```python
from build123d import *

# Parameters (mm, degrees)
BOSS_EXTRUDE1_DEPTH = 25
SKETCH2_R           = 2
CUT_EXTRUDE1_DEPTH  = 6
SKETCH3_R           = 2
CUT_EXTRUDE2_DEPTH  = 7
CUT_EXTRUDE3_START  = -7
SKETCH10_R          = 2
CUT_EXTRUDE3_DEPTH  = 7
FILLET1_R           = 15
SKETCH13_R          = 2
CUT_EXTRUDE6_DEPTH  = 156.402702679
SKETCH14_R          = 2
CUT_EXTRUDE7_DEPTH  = 92.549167118


with BuildPart() as part:
    # Sketch1 → Boss-Extrude1 (new body)
    with BuildSketch(Plane(origin=(0, 0, 0), x_dir=(1, 0, 0), z_dir=(0, 1, 0))):
        Polygon((63.5, 15), (63.5, -45), (72.5, -45), (72.5, -50), (30, -50), (30, -41), (-30, -41), (-30, -50), (-72.5, -50), (-72.5, -45), (-63.5, -45), (-63.5, 15), (-72.5, 15), (-72.5, 35), (-57.5, 35), (-57.5, -35), (57.5, -35), (57.5, 35), (72.5, 35), (72.5, 15), align=None)
    extrude(amount=BOSS_EXTRUDE1_DEPTH)

    # Sketch2 → Cut-Extrude1 (cut)
    with BuildSketch(Plane.XY.offset(41)):
        with Locations((-26.5, 12.5)):
            Circle(SKETCH2_R)
        with Locations((26.5, 12.5)):
            Circle(SKETCH2_R)
    extrude(amount=-CUT_EXTRUDE1_DEPTH, mode=Mode.SUBTRACT)

    # Sketch3 → Cut-Extrude2 (cut)
    with BuildSketch(Plane.ZY.offset(63.5)):
        with Locations((-11.5, 12.5)):
            Circle(SKETCH3_R)
        with Locations((41.5, 12.5)):
            Circle(SKETCH3_R)
    extrude(amount=-CUT_EXTRUDE2_DEPTH, mode=Mode.SUBTRACT)

    # Sketch10 → Cut-Extrude3 (cut)
    with BuildSketch(Plane(origin=(63.5, 0, 0), x_dir=(0, 0, -1), z_dir=(1, 0, 0)).offset(CUT_EXTRUDE3_START)):
        with Locations(Location((-41.5, 12.5, 0), (0, 0, 180))):
            Circle(SKETCH10_R)
        with Locations(Location((11.5, 12.5, 0), (0, 0, 180))):
            Circle(SKETCH10_R)
    extrude(amount=CUT_EXTRUDE3_DEPTH, mode=Mode.SUBTRACT)

    # Fillet1
    fillet1_edges = [part.edges().sort_by_distance(p)[0] for p in [
        (-57.5, 12.5, 35),
        (57.5, 12.5, 35),
    ]]
    fillet(fillet1_edges, radius=FILLET1_R)

    # Sketch13 → Cut-Extrude6 (cut, through all)
    with BuildSketch(Plane.ZY.offset(72.5)):
        with Locations((-30, 20)):
            Circle(SKETCH13_R)
        with Locations((-30, 5)):
            Circle(SKETCH13_R)
    extrude(amount=-CUT_EXTRUDE6_DEPTH, mode=Mode.SUBTRACT)

    # Sketch14 → Cut-Extrude7 (cut, through all)
    with BuildSketch(Plane(origin=(0, 25, 0), x_dir=(1, 0, 0), z_dir=(0, 1, 0))):
        with Locations(Location((50, -42, 0), (0, 0, 270))):
            Circle(SKETCH14_R)
        with Locations(Location((-50, -42, 0), (0, 0, 270))):
            Circle(SKETCH14_R)
    extrude(amount=-CUT_EXTRUDE7_DEPTH, mode=Mode.SUBTRACT)


solid = part.part
```
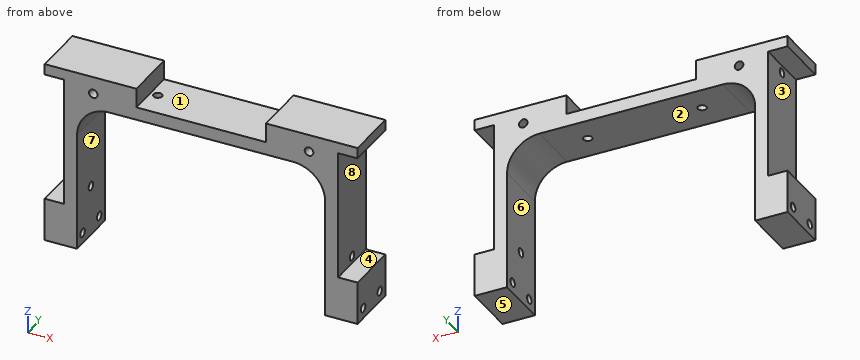
The listing builds one solid part. Answer for the finished solid, in the listing's coordinates (mm). Face numbers are marked on the shaded views. A direction names the side the tool comes from. Coordinates: 2 decimals unless noted, no trailing zeros. Write each loop counter-clockwise with the first axis right and the second up, starting at its lowest first coordinate (ties: lowest second). Pieces come first, ordered by that corner, then holes. Notation, with made-up numbers: (78.25, 42) - (120.25, 42) arc R23 ccw to (120.25, 77) - close; hole circle Ø2 at (66.25, 47). An arc over 180 degrees is marked (long way). One line per item, written item: value.
1) Find section D-D (z = 13). Give the vertices of the cut face in (x, y), and give its area (3 significant figures).
Geometry check:
outline: (-63.5, 0) - (-57.5, 0) - (-57.5, 25) - (-63.5, 25) - close; (57.5, 0) - (63.5, 0) - (63.5, 25) - (57.5, 25) - close
area: 300 mm2
2) Find section B-B (x = -26.5). Give the vertices of the cut face in (y, z).
Geometry check:
outline: (0, 35) - (10.5, 35) - (10.5, 41) - (0, 41) - close; (14.5, 35) - (25, 35) - (25, 41) - (14.5, 41) - close
3) Each of these flat-tipped pins is pushed along its axis until it touches: pin 1 Ø5 at (y, z) = (12.5, 41.5) entering from +X; pin 2 Ø3 at (y, z) = (12, 42) entering from -X; pin 3 Ø3 at (x, y) = (-1, 2.5) entering from -Z. Where does it stop, or does it pass through?
Geometry check:
pin 1: stops at x = 63.5
pin 2: stops at x = -63.5
pin 3: stops at z = 35
4) A tool of negligible diameter and unlimited length cuts with its end or side. For the marked faces 1, 2, 3 and 4, from which of +Z, -Z, +X, -X, +Y, -Y can it reach the whole face along a straight path? Write none if from no direction.
Geometry check:
face 1: +Z, +Y, -Y
face 2: -Z, +Y, -Y
face 3: -X, +Y, -Y
face 4: +X, +Y, -Y
5) For a pull along X with two mould halves and no side action, classify the marked faces 5, 6, 7 and 8 as pulls with the +X half, pulls with the -X half, needs draft (parallel to the pull), parting line crosses it, or undercut.
Geometry check:
face 5: needs draft
face 6: undercut
face 7: undercut
face 8: pulls with the +X half
6) Find section C-C (z = -11.5). Give the vertices of the cut face in (x, y).
Geometry check:
outline: (-63.5, 0) - (-57.5, 0) - (-57.5, 10.5) - (-63.5, 10.5) - close; (-63.5, 14.5) - (-57.5, 14.5) - (-57.5, 25) - (-63.5, 25) - close; (57.5, 0) - (63.5, 0) - (63.5, 10.5) - (57.5, 10.5) - close; (57.5, 14.5) - (63.5, 14.5) - (63.5, 25) - (57.5, 25) - close
7) Consider line 1 along Z through (x, y) = (59.35, 12.5); line 2 along Y through (x, z) = (66, -30); line 3 along X through (y, z) = (12.25, 42). Determine where each line is inside the solid, lowest interval first. Write a range as from..to.
Geometry check:
line 1: z = -35..-13.5, -9.5..39.5, 43.5..50
line 2: y = 0..3, 7..18, 22..25
line 3: x = -56.5..-52, -48..-30, 30..48, 52..56.5
8) Find section A-A (y = 5). Count the separate pieces of the cut face and the enclosed holes in it, and give its area (3 significant figures).
Geometry check:
separate pieces: 3
enclosed holes: 2
area: 2,610 mm2
